The drawing under review shows one solid part. Ordinate dimensions are in mm from its lowest x, y, z. Round coordinates to 2 decimals unless told otherwise and drop trailing zeros. Write each loop counter-clockwise with the first axis right and the second up, starting at its lowest first coordinate (ties: lowest second). Pieces come first, ordered by that corner, then holes. Notation, with made-up numbers: (9.25, -3.75) -> (29.25, -3.75) arc R21 ccw to (29.25, 4.25) -> close; hole circle Ø8 at (9, 82). An arc over 180 degrees is marked (long way). Answer in a Markdown table with one row per item.
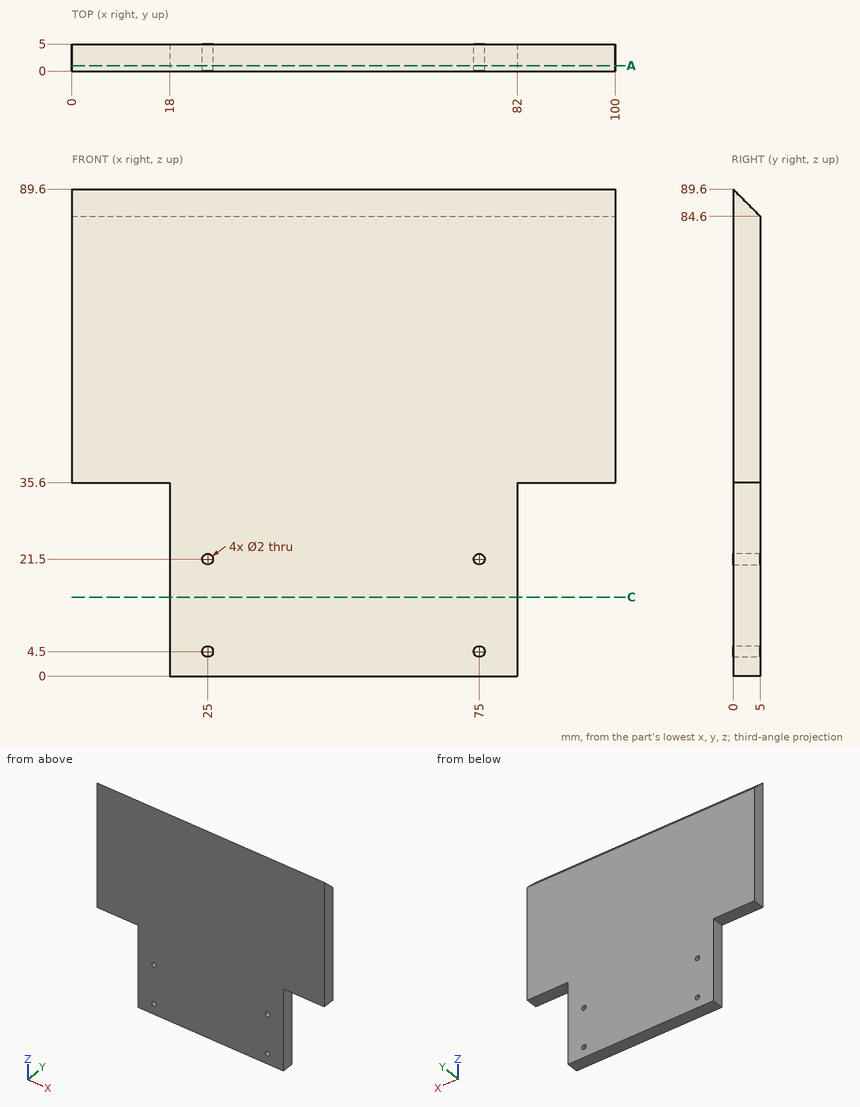
1) Clearance check with flat-ended pins moving along their axes: pin 1 Ø1.5 at (x, y) = (87.5, 2) entering from -Z; pin 2 Ø12 at (x, z) = (88.5, 21.5) entering from +Y; pin 3 Ø1 at (x, z) = (20, 15.5) entering from -Y; pin 4 Ø1.5 at (y, z) = (3.5, 15.5) entering from -X. State where each tip first meets the part, or that it passes through.
Solved:
| item | result |
|---|---|
| pin 1 | z = 35.6 |
| pin 2 | through |
| pin 3 | y = 0 |
| pin 4 | x = 18 |
2) For line 1 (X direction, y = 3.25, z = 21.5); line 2 (Z direction, x = 75, y = 1.55); line 3 (X direction, y = 1.75, z = 14), list the stretches that pass through material, from the lowest coordinate up. Write a range as [from, to].
Solved:
| item | result |
|---|---|
| line 1 | [18, 24], [26, 74], [76, 82] |
| line 2 | [0, 3.5], [5.5, 20.5], [22.5, 88.05] |
| line 3 | [18, 82] |
3) Consider section C-C on z = 14.5. State the section outline as (x, y) points, then the cut area to 3 significant figures.
Solved:
| item | result |
|---|---|
| outline | (18, 0) -> (82, 0) -> (82, 5) -> (18, 5) -> close |
| area | 320 mm² |
4) Consider section A-A on y = 1. State the section outline as (x, z) points.
Solved:
| item | result |
|---|---|
| outline | (0, 35.6) -> (18, 35.6) -> (18, 0) -> (82, 0) -> (82, 35.6) -> (100, 35.6) -> (100, 88.6) -> (0, 88.6) -> close; hole circle Ø2 at (25, 4.5); hole circle Ø2 at (25, 21.5); hole circle Ø2 at (75, 4.5); hole circle Ø2 at (75, 21.5) |
